Check sheet for the drawn part. Datum: minimum x, y, z corner. Units: mm. A direction names the side the tool comes from. Give positions to 0.01 mm unless a question says otherwise; leave off trailing zeros. Write each loop counter-clockwise with the first axis right and the second up, starting at its lowest first coordinate (ties: lowest second). Pieces come first, ordered by that corner, then holes. Notation, with made-up numbers: M 38.5,72 L 90.5,72 A26 ccw 90.5,86 Z; hole C 23,78.25 d4. An arc over 180 degrees is marked long. Use CSV: the item, a comma, the result in double quotes. Start each with the question number.
1. Access from +Z, -Z, +X, -X, +Y, -Y to the whole of each face (thin tool, end or side, straight path). Record for the marked faces 1 and 2.
2. Depth check by flat-ended pin: P1, Ø4, axis at y = 274, z = 87, coming from the +X side; P2, Ø10, axis at x = 183, z = 111.5, coming from the +Y side. Enter the tip coordinate at first touch or a pass-through.
3. Scan line: line 1 (X direction, y = 150.5, z = 81). Record every from-to range of solid material in increasing order.
4. Cross-section at A-A, the plane z = 37. Enter the section's corners in (x, y).
5. Cross-section at B-B, the plane x = 206. Enter the section's corners in (y, z).
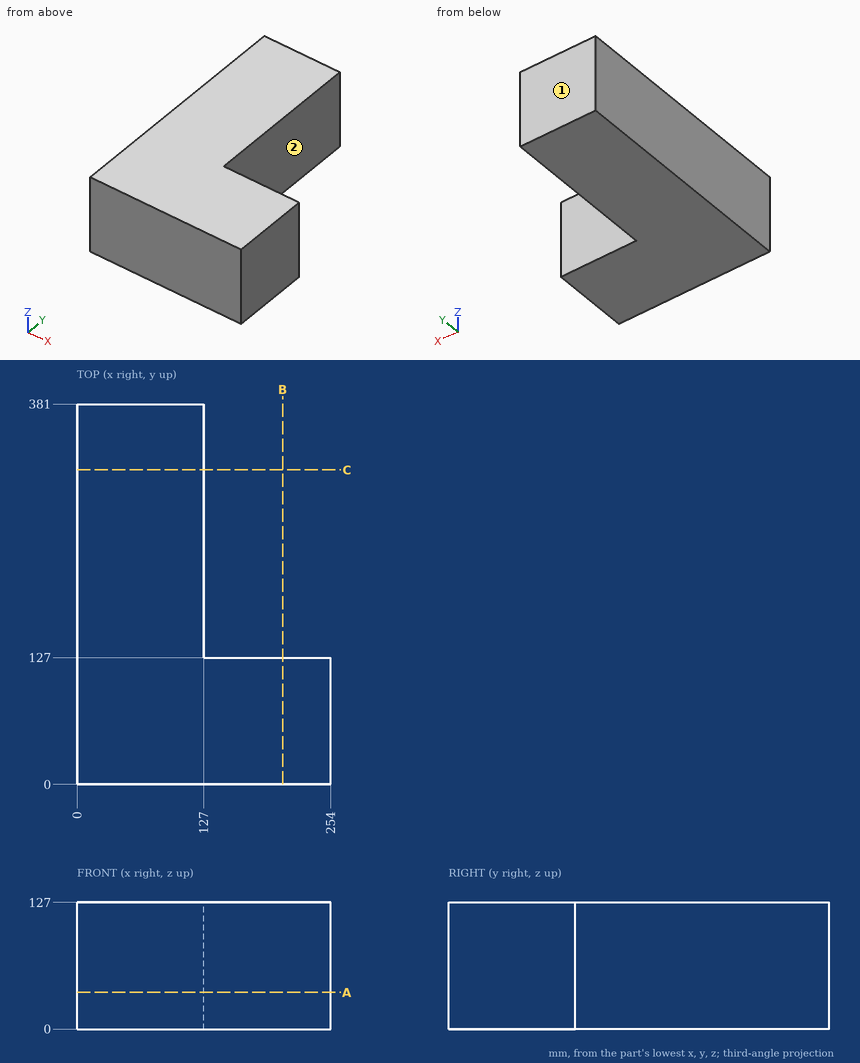
Worked answers:
1,face 1,"+Z, -Z, +X, -X, +Y"
1,face 2,"+Z, -Z, +X, +Y"
2,P1,"stops at x = 127"
2,P2,"stops at y = 127"
3,line 1,"x = 0 to 127"
4,outline,"M 0,0 L 254,0 L 254,127 L 127,127 L 127,381 L 0,381 Z"
5,outline,"M 0,0 L 127,0 L 127,127 L 0,127 Z"
